from build123d import *

# Parameters (mm, degrees)
SKETCH1_W           = 27.0002
SKETCH1_H           = 36.322
BOSS_EXTRUDE1_DEPTH = 2.3876
SKETCH2_R           = 11.9126
BOSS_EXTRUDE2_DEPTH = 28.1686
SKETCH3_R           = 10.6426
CUT_EXTRUDE1_DEPTH  = 28.1686
CUT_EXTRUDE2_REACH  = 56.608
SKETCH4_R           = 1.7272
CHAMFER1_SIZE       = 1.1303
CHAMFER1_SIZE2      = 0.158853305


with BuildPart() as part:
    # Sketch1 → Boss-Extrude1 (new body)
    with BuildSketch(Plane.XY):
        with Locations((13.5001, 18.161)):
            Rectangle(SKETCH1_W, SKETCH1_H)
    extrude(amount=BOSS_EXTRUDE1_DEPTH)

    # Sketch2 → Boss-Extrude2 (add)
    with BuildSketch(Plane.XY.offset(2.3876)):
        with Locations(Location((13.5001, 18.161, 0), (0, 0, 180))):
            Circle(SKETCH2_R)
    extrude(amount=BOSS_EXTRUDE2_DEPTH)

    # Sketch3 → Cut-Extrude1 (cut)
    with BuildSketch(Plane(origin=(0, 0, 0), x_dir=(-1, 0, 0), z_dir=(0, 0, -1))):
        with Locations((-13.5001, 18.161)):
            Circle(SKETCH3_R)
    extrude(amount=-CUT_EXTRUDE1_DEPTH, mode=Mode.SUBTRACT)

    # Sketch4 → Cut-Extrude2 (cut, up to next)
    with BuildSketch(Plane(origin=(0, 0, 0), x_dir=(-1, 0, 0), z_dir=(0, 0, -1)), mode=Mode.PRIVATE) as cut_extrude2_sk1:
        with Locations((-21.8313, 31.242)):
            Circle(SKETCH4_R)
    cut_extrude2_tool1 = extrude(cut_extrude2_sk1.sketch, amount=-CUT_EXTRUDE2_REACH, mode=Mode.PRIVATE) & part.part
    # Sketch4 → Cut-Extrude2 (cut, up to next)
    with BuildSketch(Plane(origin=(0, 0, 0), x_dir=(-1, 0, 0), z_dir=(0, 0, -1)), mode=Mode.PRIVATE) as cut_extrude2_sk2:
        with Locations((-5.1689, 5.08)):
            Circle(SKETCH4_R)
    cut_extrude2_tool2 = extrude(cut_extrude2_sk2.sketch, amount=-CUT_EXTRUDE2_REACH, mode=Mode.PRIVATE) & part.part
    add(cut_extrude2_tool1.solids().sort_by_distance((21.8313, 31.242, 0))[0], mode=Mode.SUBTRACT)
    add(cut_extrude2_tool2.solids().sort_by_distance((5.1689, 5.08, 0))[0], mode=Mode.SUBTRACT)

    # Chamfer1
    chamfer1_edges = [part.edges().sort_by_distance(p)[0] for p in [
        (23.5585, 31.242, 0),
        (6.8961, 5.08, 0),
    ]]
    chamfer1_side = [part.faces().sort_by_distance(p)[0] for p in [
        (13.5001, 0.452581317, 0),
    ]]
    chamfer(chamfer1_edges, length=CHAMFER1_SIZE, length2=CHAMFER1_SIZE2, reference=chamfer1_side[0])


solid = part.part
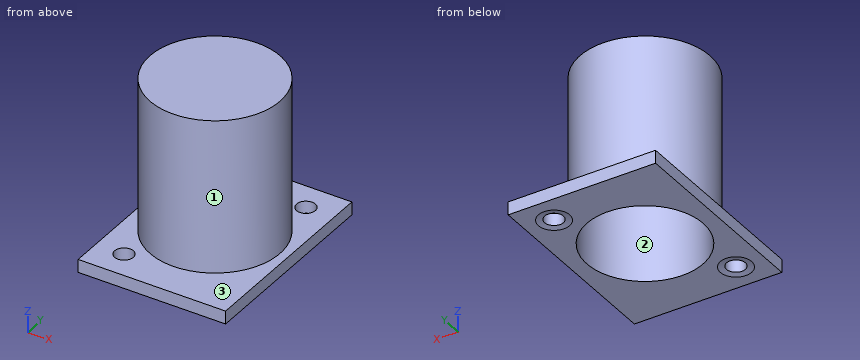
Input: part model. Units: mm. Frame: model coordinates. Face numbers are marked on the shaded views. Coordinates: 2 decimals unless noted, no trailing zeros. Write each loop counter-clockwise with the first axis right and the second up, starting at its lowest first coordinate (ties: lowest second). Pieces come first, ordered by that corner, then holes. Notation, with made-up numbers: M 8.5,37 L 35.5,37 A20 cw 35.5,49 Z; hole C 78.5,59 d4. An arc over 180 degrees is marked long. Answer as a JSON object with one key per item and string values. Group by question number.
(1) Section D-D on z = 15.5. Output: boundary loops of the cut face in (x, y), plus the area to 3 significant figures.
(2) Ray query, line 1 along Z through (x, y) = (4.25, 34); line 2 along X through (y, z) = (5, 1); line 3 along Z through (x, y) = (20.5, 12). Return the intervals inside material, ascending. Write a range as [from, to].
(3) Section A-A on y = 5.08. Output: boundary loops of the cut face in (x, z), plus the area to 3 significant figures.
(4) Contact query for flat-ended pins moving along their axis: P1, Ø1.5, axis at y = 28.5, z = 21.5, coming from the +X side; P2, Ø4.5, axis at x = 5.17, y = 5.08, coming from the -Z side; P3, Ø12, axis at y = 27, z = 15, coming from the -X side. Output: stop coordinate, or through.
(5) Section B-B on y = 10. Output: boundary loops of the cut face in (x, z), plus the area to 3 significant figures.
(6) Section C-C on x = 9.75. Output: boundary loops of the cut face in (y, z), plus the area to 3 significant figures.
(7) Mould query, pull axis X, two halves, no side actions, for the marked faces 1, 2 and 3. Classes: pulls with the +X half, pulls with the -X half, needs draft (parallel to the pull), parting line crosses it, or undercut.
Result set:
{
 "1": {"outline": "C 13.5,18.16 d23.83; hole C 13.5,18.16 d21.29", "area": "90.0 mm2"},
 "2": {"line 1": "z = [0, 2.39]", "line 2": "x = [0, 3.44], [6.89, 27]", "line 3": "z = [28.17, 30.56]"},
 "3": {"outline": "M 0,0 L 2.31,0 L 3.44,0.16 L 3.44,2.39 L 0,2.39 Z; M 6.9,0.16 L 8.03,0 L 27,0 L 27,2.39 L 6.9,2.39 Z", "area": "56.0 mm2"},
 "4": {"P1": "stops at x = 20.57", "P2": "stops at z = 0.09", "P3": "stops at x = 1.93"},
 "5": {"outline": "M 0,0 L 6.67,0 L 6.67,28.17 L 20.33,28.17 L 20.33,0 L 27,0 L 27,2.39 L 22.18,2.39 L 22.18,30.56 L 4.82,30.56 L 4.82,2.39 L 0,2.39 Z", "area": "169 mm2"},
 "6": {"outline": "M 0,0 L 8.2,0 L 8.2,28.17 L 28.12,28.17 L 28.12,0 L 36.32,0 L 36.32,2.39 L 29.47,2.39 L 29.47,30.56 L 6.85,30.56 L 6.85,2.39 L 0,2.39 Z", "area": "163 mm2"},
 "7": {"face 1": "parting line crosses it", "face 2": "undercut", "face 3": "needs draft"}
}
